CAD build for the part. Positions are in the model's coordinates, mm. Face numbers are marked on the shaded views. A direction names the side the tool comes from. Round coordinates to 2 decimals unless told otherwise and drop trailing zeros. Write each loop counter-clockwise with the first axis right and the second up, starting at its lowest first coordinate (ties: lowest second). Pieces come first, ordered by that corner, then holes. Notation, with made-up numbers: (70, -35.5) - (76, -35.5) arc R31 ccw to (76, -5.5) - close; hole circle Ø11 at (28, 23). An arc over 180 degrees is marked (long way). Answer in a Markdown table with one row per item.
Autodesk Inventor part; units mm, degrees
ref_plane "YZ Plane" through (0, 0, 0) normal (1, 0, 0) x (0, 1, 0)
ref_plane "XZ Plane" through (0, 0, 0) normal (0, 1, 0) x (-1, 0, 0)
ref_plane "XY Plane" through (0, 0, 0) normal (0, 0, 1) x (1, 0, 0)
sketch "Sketch1" plane through (0, 0, 0) normal (0, 0, 1) x (1, 0, 0)
  circle A0 centre (0, 0) radius 17.5
  arc A1 (7.4068, -21.2459) -> (7.4068, 21.2459) centre (0, 0) ccw
  arc A2 (6.0901, 17.4689) -> (6.0901, -17.4689) centre (0, 0) ccw
  line L0 (5.7609, 21.75) -> (5.7609, 16.5246) construction
  line L1 (5.7609, -16.5246) -> (5.7609, -21.75) construction
  line L2 (6.0901, -17.4689) -> (7.4068, -21.2459)
  line L3 (6.0901, 17.4689) -> (7.4068, 21.2459)
  dimension "d0" = 35
  dimension "d1" = 45
  dimension "d2" = 43.5
  dimension "d3" = 37
  dimension "d4" = 1.646
  dimension "d5" = 0.5041
  dimension "d6" = 1.646
  dimension "d7" = 0.5041
extrude "Extrusion1" add sketch "Sketch1" along normal blind 28
properties part number "PG35LHeatSink"
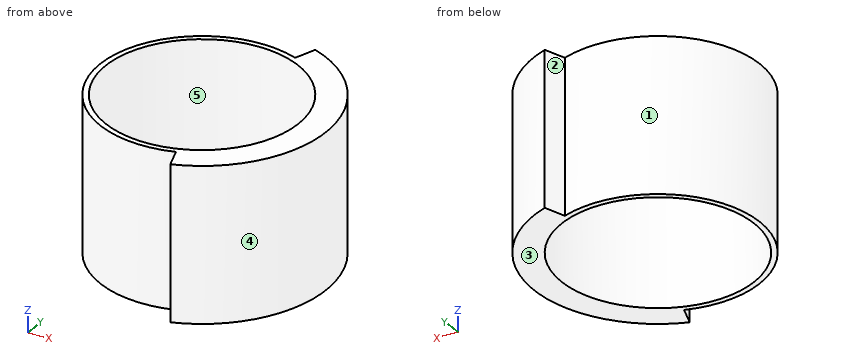
Q1. Flat gauge pins, fed straight in: pin 1 (6 mm diameter, centred on x = -8, z = 20, fed in from -Y); pin 2 (1 mm diameter, centred on x = 14, z = 4, fed in from +Y); pin 3 (8 mm diameter, centred on y = 5, z = 7, fed in from -X). Where does each tip first touch, or does it go through?
Computed:
| item | result |
|---|---|
| pin 1 | stops at y = -17.81 |
| pin 2 | stops at y = 18 |
| pin 3 | stops at x = -18.47 |
Q2. Drill centre lines: line 1 (Y direction, x = 0, z = 11.75); line 2 (X direction, y = -3, z = 14); line 3 (Y direction, x = -4, z = 7.5). Where is each one in solid material? Low to high.
Computed:
| item | result |
|---|---|
| line 1 | y = -18.5 to -17.5, 17.5 to 18.5 |
| line 2 | x = -18.26 to -17.24, 17.24 to 22.3 |
| line 3 | y = -18.06 to -17.04, 17.04 to 18.06 |
Q3. Saw through at A-A on y = 0. List the corners of the cut face in (x, z), then the cut area to 3 significant figures.
Computed:
| item | result |
|---|---|
| outline | (-18.5, 0) - (-17.5, 0) - (-17.5, 28) - (-18.5, 28) - close; (17.5, 0) - (22.5, 0) - (22.5, 28) - (17.5, 28) - close |
| area | 168 mm2 |
Q4. Saw through at D-D on x = 18.5. List the corners of the cut face in (y, z).
Computed:
| item | result |
|---|---|
| outline | (-12.81, 0) - (12.81, 0) - (12.81, 28) - (-12.81, 28) - close |
Q5. 3-axis set-ups, long thin cutter, end or side, ignore diameter. For the marked faces 1 and 2: which of +Z, -Z, +X, -X, +Y, -Y reach the whole face in a straight line?
Computed:
| item | result |
|---|---|
| face 1 | +Z, -Z |
| face 2 | +Z, -Z, +Y |
Q6. Saw through at C-C on z = 3.25. List the corners of the cut face in (x, y).
Computed:
| item | result |
|---|---|
| outline | (6.09, -17.47) - (7.41, -21.25) arc R22.5 ccw to (7.41, 21.25) - (6.09, 17.47) arc R18.5 ccw (long way) to start; hole circle Ø35 at (0, 0) |
Q7. Saw through at B-B on x = 9.5. List the corners of the cut face in (y, z).
Computed:
| item | result |
|---|---|
| outline | (-20.4, 0) - (-14.7, 0) - (-14.7, 28) - (-20.4, 28) - close; (14.7, 0) - (20.4, 0) - (20.4, 28) - (14.7, 28) - close |
Q8. Pull direction X, two halves, no side cores. Call the marked faces 3, 4 and 5: released by +X, released by -X, zero draft, split by the parting line, or undercut.
Computed:
| item | result |
|---|---|
| face 3 | zero draft |
| face 4 | released by +X |
| face 5 | undercut |
